Here's the drawing with two shaded views (mm, measured from the low corner). I have some questions. Coordinates: 2 decimals unless noted, no trailing zeros. Loops run counter-clockwise (first coordinate to the right, second up) from the corner with the lowest first, then second, coordinate; pieces in that order, holes last. Notation, with made-up numbers: (-21, 54.25) - (6, 54.25) arc R12 ccw to (6, 75.25) - close; hole circle Ø3 at (-39.5, 13.5). An arc over 180 degrees is marked (long way). One line per item, written item: value. Start each with the question number.
(1) If we section it at D-D on z = 263: Write out the boundary of the cut face in (x, y), then the cut area to 3 significant figures.
(2) I'm going to push flat-ended pins straight in: P1, Ø4, axis at x = 45.5, z = 403.5, coming from the +Y side; P2, Ø12, axis at y = 21.5, z = 169, coming from the -X side; P3, Ø1.5, axis at x = 86.5, y = 9, coming from the +Z side. Where does each tip first touch, or does it pass through?
(3) If we section it at A-A on y = 7.5: Write out the boundary of the cut face in (x, z) (1 decimal).
(4) If I drill on line 1 along X through (y, z) = (20, 300.5); line 2 along X through (y, z) = (12.25, 300) (1 decimal); line 3 along Y through (x, z) = (17.5, 337.5), over which ranges is the centre line in solid material (lowest first)? Write a range as from..to.
(5) If we section it at B-B on x = 89.5: Write out the boundary of the cut face in (y, z) (1 decimal).
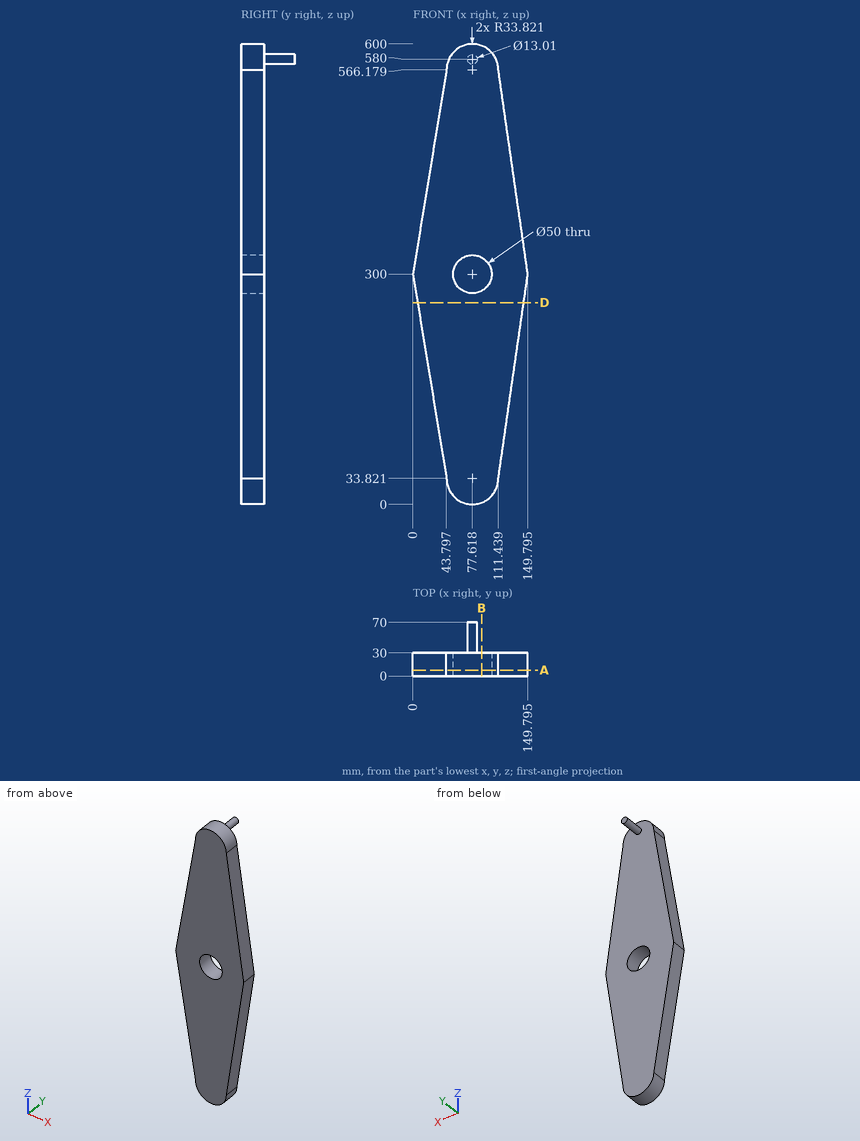
Values:
1. outline: (6.09, 0) - (144.46, 0) - (144.46, 30) - (6.09, 30) - close
1. area: 4,150 mm2
2. P1: stops at y = 30
2. P2: stops at x = 20.57
2. P3: stops at z = 599.01
3. outline: (0, 300) - (43.8, 33.8) arc R33.8 ccw to (111.4, 33.8) - (149.8, 300) - (111.4, 566.2) arc R33.8 ccw to (43.8, 566.2) - close; hole circle Ø50 at (77.6, 300)
4. line 1: x = 0.08..52.62, 102.61..149.72
4. line 2: x = 0..52.6, 102.6..149.8
4. line 3: y = 0..30
5. outline: (0, 2.2) - (30, 2.2) - (30, 278) - (0, 278) - close; (0, 322) - (30, 322) - (30, 597.8) - (0, 597.8) - close
